```python
from build123d import *

# Parameters (mm, degrees)
SKETCH_1_W          = 20
SKETCH_1_H          = 20
SKETCH_1_W_2        = 18
SKETCH_1_H_2        = 18
EXTRUDE_1_DEPTH     = 460
SKETCH_2_R          = 1.8
CUT_EXTRUDE_1_DEPTH = 3
SKETCH_3_R          = 1.8
CUT_EXTRUDE_2_DEPTH = 3
SKETCH_5_R          = 1.8
CUT_EXTRUDE_3_DEPTH = 3
SKETCH_6_R          = 1.8
CUT_EXTRUDE_4_DEPTH = 10
SKETCH_7_R          = 1.5
CUT_EXTRUDE_5_DEPTH = 20
SKETCH1_R           = 2.5
CUT_EXTRUDE1_DEPTH  = 20
SKETCH2_R           = 2.6
CUT_EXTRUDE2_DEPTH  = 36


with BuildPart() as part:
    # 草图1 → 凸台-拉伸1 (new body)
    with BuildSketch(Plane.XY):
        Rectangle(SKETCH_1_W, SKETCH_1_H)
        Rectangle(SKETCH_1_W_2, SKETCH_1_H_2, mode=Mode.SUBTRACT)
    extrude(amount=EXTRUDE_1_DEPTH)

    # 草图2 → 切除-拉伸1 (cut)
    with BuildSketch(Plane.ZY.offset(10)):
        with Locations((10, 0)):
            Circle(SKETCH_2_R)
    extrude(amount=-CUT_EXTRUDE_1_DEPTH, mode=Mode.SUBTRACT)

    # 草图3 → 切除-拉伸2 (cut)
    with BuildSketch(Plane.ZY.offset(10)):
        with Locations((198, 0)):
            Circle(SKETCH_3_R)
    extrude(amount=-CUT_EXTRUDE_2_DEPTH, mode=Mode.SUBTRACT)

    # 草图5 → 切除-拉伸3 (cut)
    with BuildSketch(Plane.ZY.offset(10)):
        with Locations((450, 0)):
            Circle(SKETCH_5_R)
    extrude(amount=-CUT_EXTRUDE_3_DEPTH, mode=Mode.SUBTRACT)

    # 草图6 → 切除-拉伸4 (cut)
    with BuildSketch(Plane.ZY.offset(10)):
        with Locations((262, 0)):
            Circle(SKETCH_6_R)
    extrude(amount=-CUT_EXTRUDE_4_DEPTH, mode=Mode.SUBTRACT)

    # 草图7 → 切除-拉伸5 (cut)
    with BuildSketch(Plane(origin=(0, 10, 0), x_dir=(1, 0, 0), z_dir=(0, 1, 0))):
        with Locations((4, -166)):
            Circle(SKETCH_7_R)
        with Locations((-6, -166)):
            Circle(SKETCH_7_R)
        with Locations((4, -178)):
            Circle(SKETCH_7_R)
        with Locations((-6, -178)):
            Circle(SKETCH_7_R)
    extrude(amount=-CUT_EXTRUDE_5_DEPTH, mode=Mode.SUBTRACT)

    # Sketch1 → Cut-Extrude1 (cut)
    with BuildSketch(Plane.XZ.offset(10)):
        with Locations((0, 60)):
            Circle(SKETCH1_R)
    extrude(amount=-CUT_EXTRUDE1_DEPTH, mode=Mode.SUBTRACT)

    # Sketch2 → Cut-Extrude2 (cut)
    with BuildSketch(Plane.XZ.offset(10)):
        with Locations((0, 400)):
            Circle(SKETCH2_R)
    extrude(amount=-CUT_EXTRUDE2_DEPTH, mode=Mode.SUBTRACT)


solid = part.part
```
The listing builds one solid part. Answer for the finished solid, in the listing's coordinates (mm). A direction names the side the tool comes from. Give positions to 0.01 mm unless a question says otherwise; leave off trailing zeros. Loops run counter-clockwise (first coordinate to the right, second up) from the corner with the lowest first, then second, coordinate; pieces in that order, holes last. Notation, with made-up numbers: (67.5, 42) - (121.5, 42) arc R31 ccw to (121.5, 81) - close; hole circle Ø9 at (4, 44.25). An arc over 180 degrees is marked (long way). Answer as CSV lines item,"result". Start each with the question number.
Item 1: A cutting plane is placed at A-A on y = 5. Determine the outline of the cut face in (x, z), then the cut area to 3 significant figures.
Item 2: A cutting plane is placed at B-B on z = 352. Determine the outline of the cut face in (x, y).
Item 3: For faces 1 (the face through (-0.8, -9.6, 460)), 2 (the face through (-9, 0, 227)), determine the directions among +Z, -Z, +X, -X, +Y, -Y from which every point of the face is accessible in a straight line to the end or side of a thin tool.
Item 4: Find the intervals of material crossed by line 1 (Z direction, x = 0, y = -9.55); line 2 (X direction, y = -0.25, z = 308), in increasing order. Write a range as from..to.
Item 5: This flat-tipped pin is pushed along its axis until it touches: pin 1 (3 mm diameter, centred on y = 0, z = 262, fed in from -X). Where does it stop, or does it pass through?
Item 6: The mould has two halves that part along Y. Classify faces 3 (the face through (0, 9, 227)), 4 (the face through (-0.8, -9.6, 0)), 5 (the face through (0, 10, 227)): +Y half, -Y half, draft (parallel to the pull), parting line (faces both ways), or undercut.
Found:
1,outline,"(-10, 0) - (-9, 0) - (-9, 460) - (-10, 460) - close; (9, 0) - (10, 0) - (10, 460) - (9, 460) - close"
1,area,"920 mm^2"
2,outline,"(-10, -10) - (10, -10) - (10, 10) - (-10, 10) - close; hole (-9, -9) - (9, -9) - (9, 9) - (-9, 9) - close"
3,face 1,"+Z, +X, -X, +Y, -Y"
3,face 2,"+Z, -Z"
4,line 1,"z = 0..57.5, 62.5..397.4, 402.6..460"
4,line 2,"x = -10..-9, 9..10"
5,pin 1,"stops at x = 9"
6,face 3,"undercut"
6,face 4,"draft"
6,face 5,"+Y half"
